Could you check a few things on this model? Use its own coordinates, in mm. A direction names the side the tool comes from. Give positions to 0.01 mm unless a question says otherwise; leave off trailing zeros. Order: outer loops, then holes, each group sorted by start corner. A loop starts at its lowest first (then second) coordinate and runs counter-clockwise, first axis right, second up. Notation, with made-up numbers: (-39, 83.5) - (11, 83.5) arc R4 cw to (11, 87.5) - close; hole circle Ø5 at (86, 6.5). An arc over 180 degrees is marked (long way). Put each result on its own line as item: value.
from build123d import *

# Parameters (mm, degrees)
SKETCH_1_W          = 60
SKETCH_1_H          = 70
EXTRUDE_1_DEPTH     = 10
SKETCH_2_R          = 3
CUT_EXTRUDE_1_DEPTH = 48.16990566
CUT_EXTRUDE_START   = -4
SKETCH_3_R          = 7.5
SKETCH_3_R_2        = 3
CUT_EXTRUDE_2_DEPTH = 4
SKETCH_4_R          = 5
CUT_EXTRUDE_3_DEPTH = 1
EXTRUDE_2_DEPTH     = 12.5
SKETCH_7_R          = 9.5
CUT_EXTRUDE_4_DEPTH = 12.5
CUT_EXTRUDE_5_DEPTH = 57.5
SKETCH_9_R          = 1.5
CUT_EXTRUDE_6_DEPTH = 62.032778079
SKETCH_10_W         = 13
SKETCH_10_H         = 12.5
CUT_EXTRUDE_7_DEPTH = 13
SKETCH_11_W         = 13
SKETCH_11_H         = 12.5
CUT_EXTRUDE_8_DEPTH = 13
EXTRUDE_START       = -5
SKETCH_12_R         = 9.5
SKETCH_12_R_2       = 8
EXTRUDE_3_DEPTH     = 5


with BuildPart() as part:
    # 草图1 → 凸台-拉伸1 (new body)
    with BuildSketch(Plane.XY):
        Rectangle(SKETCH_1_W, SKETCH_1_H)
    extrude(amount=EXTRUDE_1_DEPTH)

    # 草图2 → 切除-拉伸1 (cut, through all)
    with BuildSketch(Plane.XY.offset(10)):
        with Locations((-8, 15)):
            Circle(SKETCH_2_R)
        with Locations((7, 15)):
            Circle(SKETCH_2_R)
        with Locations((-8, -15)):
            Circle(SKETCH_2_R)
        with Locations((7, -15)):
            Circle(SKETCH_2_R)
        with Locations((22, 15)):
            Circle(SKETCH_2_R)
        with Locations((22, -15)):
            Circle(SKETCH_2_R)
    extrude(amount=-CUT_EXTRUDE_1_DEPTH, mode=Mode.SUBTRACT)

    # 草图3 → 切除-拉伸2 (cut)
    # profile 1 of 2: a face of its own
    with BuildSketch(Plane(origin=(0, 0, 0), x_dir=(-1, 0, 0), z_dir=(0, 0, -1)).offset(CUT_EXTRUDE_START)):
        with Locations((8, 15)):
            Circle(SKETCH_3_R)
        with Locations(Location((8, 15, 0), (0, 0, 180))):
            Circle(SKETCH_3_R_2, mode=Mode.SUBTRACT)
    # profile 2 of 2: a face of its own
    with BuildSketch(Plane(origin=(0, 0, 0), x_dir=(-1, 0, 0), z_dir=(0, 0, -1)).offset(CUT_EXTRUDE_START)):
        with BuildLine():
            ThreePointArc((8, 7.5), (0.5, 15), (8, 22.5))
            Line((8, 22.5), (-30, 22.5))
            Line((-30, 22.5), (-30, 7.5))
            Line((-30, 7.5), (8, 7.5))
        make_face()
        with Locations(Location((-7, 15, 0), (0, 0, 180))):
            Circle(SKETCH_3_R_2, mode=Mode.SUBTRACT)
    cut_extrude_2 = extrude(amount=CUT_EXTRUDE_2_DEPTH, mode=Mode.SUBTRACT)

    # 镜向1: 切除-拉伸2 across plane
    add(cut_extrude_2.mirror(Plane.ZX), mode=Mode.SUBTRACT)

    # 草图4 → 切除-拉伸3 (cut)
    with BuildSketch(Plane.XY.offset(10)):
        with Locations((-20, 0)):
            Circle(SKETCH_4_R)
        with BuildLine():
            ThreePointArc((-20, -5), (-25, 0), (-20, 5))
            Line((-20, 5), (-30, 5))
            Line((-30, 5), (-30, -5))
            Line((-30, -5), (-20, -5))
        make_face()
    extrude(amount=-CUT_EXTRUDE_3_DEPTH, mode=Mode.SUBTRACT)

    # 草图6 → 凸台-拉伸2 (add)
    with BuildSketch(Plane(origin=(0, 35, 0), x_dir=(1, 0, 0), z_dir=(0, 1, 0))):
        with BuildLine():
            ThreePointArc((30, 0), (20.807611845, 3.807611845), (17, 13))
            ThreePointArc((17, 13), (0, 30), (-17, 13))
            ThreePointArc((-17, 13), (-20.807611845, 3.807611845), (-30, 0))
            Line((-30, 0), (30, 0))
        make_face()
    extrude_2 = extrude(amount=-EXTRUDE_2_DEPTH)

    # 草图7 → 切除-拉伸4 (cut)
    with BuildSketch(Plane(origin=(0, 35, 0), x_dir=(1, 0, 0), z_dir=(0, 1, 0))):
        with Locations(Location((0, 13, 0), (0, 0, 270))):
            Circle(SKETCH_7_R)
    cut_extrude_4 = extrude(amount=-CUT_EXTRUDE_4_DEPTH, mode=Mode.SUBTRACT)

    # 镜向2: 凸台-拉伸2, 切除-拉伸4 across plane
    add(extrude_2.mirror(Plane.ZX))
    add(cut_extrude_4.mirror(Plane.ZX), mode=Mode.SUBTRACT)

    # 草图8 → 切除-拉伸5 (cut)
    with BuildSketch(Plane.XZ.offset(35)):
        with BuildLine():
            Line((-30, 10), (-30, 0))
            ThreePointArc((-30, 0), (-20.807611845, -3.807611845), (-17, -13))
            ThreePointArc((-17, -13), (0, -30), (17, -13))
            ThreePointArc((17, -13), (20.807611845, -3.807611845), (30, 0))
            Line((30, 0), (30, 10))
            Line((30, 10), (-30, 10))
        make_face()
    extrude(amount=-CUT_EXTRUDE_5_DEPTH, mode=Mode.SUBTRACT)

    # 草图9 → 切除-拉伸6 (cut, through all)
    with BuildSketch(Plane.XY.offset(10)):
        with Locations((-24, 28.5)):
            Circle(SKETCH_9_R)
        with Locations((24, 28.5)):
            Circle(SKETCH_9_R)
    extrude(amount=-CUT_EXTRUDE_6_DEPTH, mode=Mode.SUBTRACT)

    # 草图10 → 切除-拉伸7 (cut)
    with BuildSketch(Plane(origin=(30, 0, 0), x_dir=(0, 0, -1), z_dir=(1, 0, 0))):
        with Locations((6.5, 28.75)):
            Rectangle(SKETCH_10_W, SKETCH_10_H)
    extrude(amount=-CUT_EXTRUDE_7_DEPTH, mode=Mode.SUBTRACT)

    # 草图11 → 切除-拉伸8 (cut)
    with BuildSketch(Plane.ZY.offset(30)):
        with Locations((-6.5, 28.75)):
            Rectangle(SKETCH_11_W, SKETCH_11_H)
    extrude(amount=-CUT_EXTRUDE_8_DEPTH, mode=Mode.SUBTRACT)

    # 草图12 → 凸台-拉伸3 (add)
    with BuildSketch(Plane.XZ.offset(-22.5).offset(EXTRUDE_START)):
        with Locations(Location((0, -13, 0), (0, 0, 90))):
            Circle(SKETCH_12_R)
        with Locations(Location((0, -13, 0), (0, 0, 270))):
            Circle(SKETCH_12_R_2, mode=Mode.SUBTRACT)
    extrude(amount=EXTRUDE_3_DEPTH)


solid = part.part
1) Suppose I cut it at A-A, the plane y = 28.5. List the corners of the cut face in (x, z) for me, and give its area (3 significant figures).
Filled in:
outline: (-30, 0) - (-25.5, 0) - (-25.5, 10) - (-30, 10) - close; (-22.5, 0) - (-17, 0) - (-17, -13) arc R17 ccw to (17, -13) - (17, 0) - (22.5, 0) - (22.5, 10) - (-22.5, 10) - close; (25.5, 0) - (30, 0) - (30, 10) - (25.5, 10) - close; hole circle Ø19 at (0, -13)
area: 1,150 mm^2
2) If I drill on line 1 (Y direction, x = -24, z = 6.25); line 2 (Z direction, x = 0, y = 29.25); line 3 (X direction, y = 30.25, z = -13), over which ranges is the centre line in solid material (lowest first)? Write a range as [from, to].
Filled in:
line 1: y = [22.5, 27], [30, 35]
line 2: z = [-30, -22.5], [-3.5, 10]
line 3: x = [-17, -9.5], [9.5, 17]
3) Suppose I cut it at D-D, the plane y = 24.5. List the corners of the cut face in (x, z) for me.
Filled in:
outline: (-30, 0) - (-17, 0) - (-17, -13) arc R17 ccw to (17, -13) - (17, 0) - (30, 0) - (30, 10) - (-30, 10) - close; hole circle Ø16 at (0, -13)
4) Which directions (+Z, -Z, +X, -X, +Y, -Y) give clear straight access to the entire face, cutting with the end or side of a thin tool? Please do faces 4 (the flat face through (22, 29, 0)), 5 (the cylindrical face through (22.89, 29.51, 5.07)), 6 (the cylindrical face through (0.42, 31.3, -22.49)), 7 (the flat face through (0, 35, -1)), 8 (the flat face through (-17, 29, -7)).
Filled in:
face 4: -Z, +X, +Y, -Y
face 5: +Z, -Z
face 6: +Y
face 7: +Z, -Z, +X, -X, +Y
face 8: -Z, -X, +Y, -Y
5) Suppose I cut it at B-B, the plane x = 24. List the corners of the cut face in (y, z) for me, and give its area (3 significant figures).
Filled in:
outline: (22.5, 0) - (27, 0) - (27, 10) - (22.5, 10) - close; (30, 0) - (35, 0) - (35, 10) - (30, 10) - close
area: 95.0 mm^2
6) We'd pull the mould along Y, two halves only. Please class faces 1 (the flat face through (17, 29, -6)), 2 (the flat face through (0, 22.5, -1)), 3 (the cylindrical face through (-24, 30, 5)): pulls with the +Y half, pulls with the -Y half, needs draft (parallel to the pull), parting line crosses it, or undercut.
Filled in:
face 1: needs draft
face 2: pulls with the -Y half
face 3: undercut
7) I'm going to push flat-ended pins straight in: pin 1 (18.5 mm diameter, centred on x = 0, z = -13, fed in from -Y); pin 2 (4 mm diameter, centred on y = 26, z = -14.5, fed in from -X); pin 3 (4 mm diameter, centred on x = 24.5, y = 31.5, fed in from -Z); pin 4 (4 mm diameter, centred on y = 25, z = -25.5, fed in from +X). Where does each tip first touch, or does it pass through?
Filled in:
pin 1: stops at y = 22.5
pin 2: stops at x = -17
pin 3: stops at z = 0
pin 4: stops at x = 13.37
8) Suppose I cut it at C-C, the plane z = -6. List the corners of the cut face in (x, y) for me, and give its area (3 significant figures).
Filled in:
outline: (-17, 22.5) - (-3.87, 22.5) - (-3.87, 27.5) - (-6.42, 27.5) - (-6.42, 35) - (-17, 35) - close; (3.87, 22.5) - (17, 22.5) - (17, 35) - (6.42, 35) - (6.42, 27.5) - (3.87, 27.5) - close
area: 290 mm^2
